For this review, take the finished solid that the model builds, in its own axes (mm). Face numbers are marked on the shaded views. A direction names the side the tool comes from. Coordinates: 2 decimals unless noted, no trailing zeros. Loops run counter-clockwise (first coordinate to the right, second up) from the corner with the lowest first, then second, coordinate; pieces in that order, holes last. Notation, with made-up numbers: (82, 38.25) -> (136, 38.25) arc R6 ccw to (136, 43.25) -> close; hole circle Ø7 at (45, 64.25). An arc over 180 degrees is marked (long way). Answer in a Markdown table with one row per item.
from build123d import *

# Parameters (mm, degrees)
BOSS_EXTRUDE1_DEPTH = 3.048
FILLET1_R           = 0.127


with BuildPart() as part:
    # Sketch1 → Boss-Extrude1 (new body, symmetric)
    with BuildSketch(Plane.XY):
        with BuildLine():
            ThreePointArc((0, 27.535484012), (-9.412998127, 39.802742006), (0, 52.07))
            Line((0, 52.07), (-11.040532194, 49.111698314))
            ThreePointArc((-11.040532194, 49.111698314), (-39.066320922, 14.192289272), (-14.190605813, -23.03684931))
            Line((-14.190605813, -23.03684931), (0, -28.201807432))
            ThreePointArc((0, -28.201807432), (8.35634418, -40.135903716), (0, -52.07))
            Line((0, -52.07), (10.740686656, -48.160709762))
            ThreePointArc((10.740686656, -48.160709762), (36.144496882, -10.141220984), (7.52373904, 25.519504212))
            Line((7.52373904, 25.519504212), (0, 27.535484012))
        make_face()
        with BuildLine():
            Line((-14.441907141, 2.546497882), (-6.036047045, 12.564211851))
            ThreePointArc((-6.036047045, 12.564211851), (-5.686528205, 15.219071016), (-3.428121714, 13.780307404))
            ThreePointArc((-3.428121714, 13.780307404), (-3.434162631, 13.641947663), (-3.452239406, 13.504640922))
            Line((-3.452239406, 13.504640922), (9.426285427, 11.233809522))
            Line((9.426285427, 11.233809522), (14.441907141, -2.546497882))
            Line((14.441907141, -2.546497882), (5.015621714, -13.780307404))
            Line((5.015621714, -13.780307404), (-9.426285427, -11.233809522))
            Line((-9.426285427, -11.233809522), (-14.441907141, 2.546497882))
        make_face(mode=Mode.SUBTRACT)
    extrude(amount=BOSS_EXTRUDE1_DEPTH, both=True)

    # Fillet1
    fillet1_edges = [part.edges().sort_by_distance(p)[0] for p in [
        (0, 52.07, 0),
        (0, -52.07, 0),
    ]]
    fillet(fillet1_edges, radius=FILLET1_R)


solid = part.part
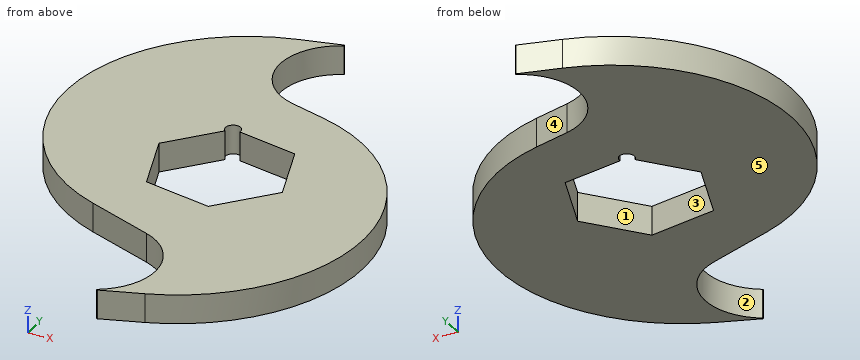
Item 1: The part is to be moulded in two halves that separate along X. For the marked faces 3, 4 and 5, say which applies: +X half, -X half, draft (parallel to the pull), parting line (faces both ways), or undercut.
Worked answers:
| item | result |
|---|---|
| face 3 | undercut |
| face 4 | +X half |
| face 5 | draft |
Item 2: Insertion check: pin 1 (1.5 mm diameter, centred on y = 30, z = -2, fed in from +X). The pin has a flat end and moves straight along its axis. Give the tip position at first contact, or say it passes through.
Worked answers:
| item | result |
|---|---|
| pin 1 | x = -3.78 |
Item 3: Take a section at B-B, the plane x = 12. State the section outline as (y, z) points.
Worked answers:
| item | result |
|---|---|
| outline | (-47.68, -3.05) -> (-5.46, -3.05) -> (-5.46, 3.05) -> (-47.68, 3.05) -> close; (4.16, -3.05) -> (24.02, -3.05) -> (24.02, 3.05) -> (4.16, 3.05) -> close |
Item 4: Take a section at C-C, the plane y = 17.5. State the section outline as (x, z) points.
Worked answers:
| item | result |
|---|---|
| outline | (-38.78, -3.05) -> (22.71, -3.05) -> (22.71, 3.05) -> (-38.78, 3.05) -> close |
Item 5: Take a section at A-A, the plane y = -1. State the section outline as (x, z) points, and give its area (3 significant figures).
Worked answers:
| item | result |
|---|---|
| outline | (-36.6, -3.05) -> (-13.15, -3.05) -> (-13.15, 3.05) -> (-36.6, 3.05) -> close; (13.88, -3.05) -> (34.63, -3.05) -> (34.63, 3.05) -> (13.88, 3.05) -> close |
| area | 269 mm² |
Item 6: For the marked faces 1 and 2, list the 3-axis set-ups (+Z, -Z, +X, -X, +Y, -Y) from which the entire face can be reached by the end or side of a thin tool; tool diameter is ignored.
Worked answers:
| item | result |
|---|---|
| face 1 | +Z, -Z |
| face 2 | +Z, -Z, -X |
Item 7: For L1, parallel to Y at x = 5.5, z = -2.5; L2, parallel to Y at x = -36, z = -2; L3, parallel to X at y = 6.5, z = 1, list the stretches that pass through material, from the lowest coordinate up.
Worked answers:
| item | result |
|---|---|
| L1 | -50.07 to -48.16, -32.11 to -13.2, 11.93 to 26.06 |
| L2 | -2.47 to 27.55 |
| L3 | -38.62 to -11.12, 11.15 to 31.56 |
Item 8: Take a section at D-D, the plane y = -22. State the section outline as (x, z) points.
Worked answers:
| item | result |
|---|---|
| outline | (-16.75, -3.05) -> (34.82, -3.05) -> (34.82, 3.05) -> (-16.75, 3.05) -> close |
